from build123d import *

# Parameters (mm, degrees)
SKETCH_1_W          = 250
SKETCH_1_H          = 220.8
EXTRUDE_1_DEPTH     = 3
CUT_EXTRUDE_1_REACH = 223.019
SKETCH_2_W          = 30
SKETCH_2_H          = 10
SKETCH_3_R          = 1.5
CUT_EXTRUDE_2_DEPTH = 295.913282021


with BuildPart() as part:
    # 草图1 → 凸台-拉伸1 (new, symmetric)
    with BuildSketch(Plane(origin=(0, 0, 0), x_dir=(1, 0, 0), z_dir=(0, 1, 0))):
        with Locations((31.040268456, -46.012416107)):
            Rectangle(SKETCH_1_W, SKETCH_1_H)
    extrude(amount=EXTRUDE_1_DEPTH, both=True)

    # 草图2 → 切除-拉伸1 (cut, up to next)
    with BuildSketch(Plane(origin=(0, 3, 0), x_dir=(1, 0, 0), z_dir=(0, 1, 0)), mode=Mode.PRIVATE) as cut_extrude_1_sk1:
        with Locations((-42.959731544, -151.412416107)):
            Rectangle(SKETCH_2_W, SKETCH_2_H)
    cut_extrude_1_tool1 = extrude(cut_extrude_1_sk1.sketch, amount=-CUT_EXTRUDE_1_REACH, mode=Mode.PRIVATE) & part.part
    # 草图2 → 切除-拉伸1 (cut, up to next)
    with BuildSketch(Plane(origin=(0, 3, 0), x_dir=(1, 0, 0), z_dir=(0, 1, 0)), mode=Mode.PRIVATE) as cut_extrude_1_sk2:
        with Locations((31.040268456, -151.412416107)):
            Rectangle(SKETCH_2_W, SKETCH_2_H)
    cut_extrude_1_tool2 = extrude(cut_extrude_1_sk2.sketch, amount=-CUT_EXTRUDE_1_REACH, mode=Mode.PRIVATE) & part.part
    # 草图2 → 切除-拉伸1 (cut, up to next)
    with BuildSketch(Plane(origin=(0, 3, 0), x_dir=(1, 0, 0), z_dir=(0, 1, 0)), mode=Mode.PRIVATE) as cut_extrude_1_sk3:
        with Locations((105.040268456, -151.412416107)):
            Rectangle(SKETCH_2_W, SKETCH_2_H)
    cut_extrude_1_tool3 = extrude(cut_extrude_1_sk3.sketch, amount=-CUT_EXTRUDE_1_REACH, mode=Mode.PRIVATE) & part.part
    add(cut_extrude_1_tool1.solids().sort_by_distance((-42.959732, 3, 151.412416))[0], mode=Mode.SUBTRACT)
    add(cut_extrude_1_tool2.solids().sort_by_distance((31.040268, 3, 151.412416))[0], mode=Mode.SUBTRACT)
    add(cut_extrude_1_tool3.solids().sort_by_distance((105.040268, 3, 151.412416))[0], mode=Mode.SUBTRACT)

    # 草图3 → 切除-拉伸2 (cut, through all)
    with BuildSketch(Plane.ZY.offset(93.959731544)):
        with Locations((153.412416107, 0)):
            Circle(SKETCH_3_R)
        with BuildLine():
            Line((156.412416107, 3), (153.412416107, 3))
            ThreePointArc((153.412416107, 3), (155.533736451, 2.121320344), (156.412416107, 0))
            Line((156.412416107, 0), (156.412416107, 3))
        make_face()
        with BuildLine():
            Line((156.412416107, -3), (156.412416107, 0))
            ThreePointArc((156.412416107, 0), (155.533736451, -2.121320344), (153.412416107, -3))
            Line((153.412416107, -3), (156.412416107, -3))
        make_face()
    extrude(amount=-CUT_EXTRUDE_2_DEPTH, mode=Mode.SUBTRACT)


solid = part.part
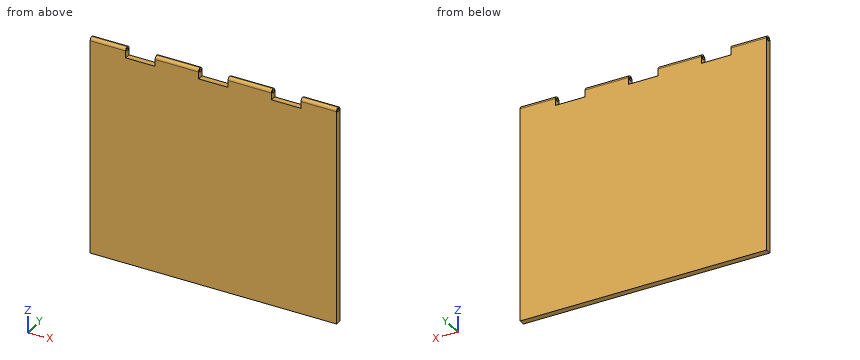
Geometry: final body of the model. Coordinates: model frame, mm. Coordinates: 2 decimals unless noted, no trailing zeros. Loops run counter-clockwise (first coordinate to the right, second up) from the corner with the lowest first, then second, coordinate; pieces in that order, holes last. Notation, with made-up numbers: M 8.5,-16 L 52.5,-16 A19 ccw 52.5,-5 Z; hole C -1.75,17 d9. An arc over 180 degrees is marked long. One line per item, written item: value. Start each with the question number.
1) Pin query (flat end, axial travel): P1, Ø1, axis at x = 102, y = -0.5, coming from the +Z side. Return the tip coordinate at first contact, or that it passes through.
2) Material intervals for L1, parallel to Z at x = 27.5, y = -2.25; L2, parallel to Z at x = -60, y = 1.25; L3, parallel to Z at x = -23, y = -0.5, sorted ascending. Write a range as from..to.
3) Cut plane A-A (x = -36.5). Return loops of the section in (y, z).
Evaluation:
1. P1: z = 146.41
2. L1: -64.39..146.41
2. L2: -64.39..152.58, 154.24..156.14
2. L3: -64.39..152, 154.83..156.37
3. outline: M -3,-64.39 L 3,-64.39 L 3,146.41 L -3,146.41 Z
